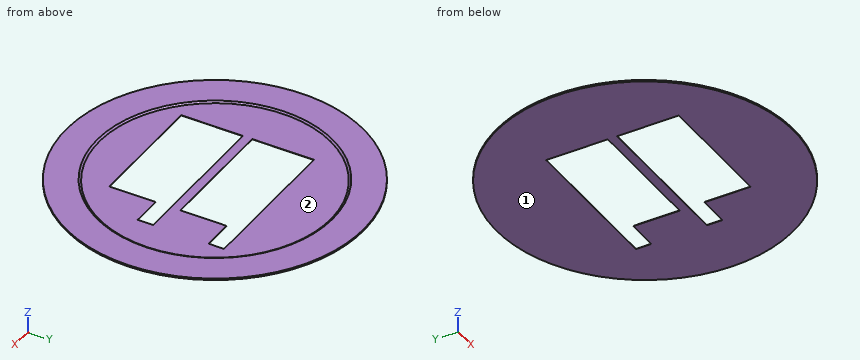
```python
from build123d import *

# Parameters (mm, degrees)
SKETCH3_W          = 40
SKETCH3_H          = 20
SKETCH3_W_2        = 10
SKETCH3_H_2        = 5
CUT_EXTRUDE1_DEPTH = 69.156113896


with BuildPart() as part:
    # Sketch2 → Revolve1 (revolve)
    with BuildSketch(Plane.YZ, mode=Mode.PRIVATE) as revolve1_sk:
        Polygon((48.192820323, 0.5), (38.192820323, 0.5), (37.5, 0.1), (0, 0.1), (0, 0), (48.192820323, 0), align=None)
    revolve(revolve1_sk.sketch.rotate(Axis((0, 0, 0.1), (0, 0, -1)), 90), axis=Axis((0, 0, 0.1), (0, 0, -1)))

    # Sketch3 → Cut-Extrude1 (cut, through all)
    with BuildSketch(Plane.XY.offset(0.1)):
        with Locations((-2.605575449, 8.919047288)):
            Rectangle(SKETCH3_W, SKETCH3_H)
        with Locations((22.394424551, 16.419047288)):
            Rectangle(SKETCH3_W_2, SKETCH3_H_2)
        with Locations((-2.605575449, -14.080952712)):
            Rectangle(SKETCH3_W, SKETCH3_H)
        with Locations((22.394424551, -6.580952712)):
            Rectangle(SKETCH3_W_2, SKETCH3_H_2)
    extrude(amount=-CUT_EXTRUDE1_DEPTH, mode=Mode.SUBTRACT)


solid = part.part
```
The listing builds one solid part. Answer for the finished solid, in the listing's coordinates (mm). Face numbers are marked on the shaded views. Coordinates: 2 decimals unless noted, no trailing zeros. Loops run counter-clockwise (first coordinate to the right, second up) from the corner with the lowest first, then second, coordinate; pieces in that order, holes last. Notation, with made-up numbers: (4.5, -15.5) - (40.5, -15.5) arc R12 ccw to (40.5, -1.5) - close; hole circle Ø10 at (61.5, 24). An arc over 180 degrees is marked (long way). Use a Markdown table: item, result. Add a question column.
1) The mould has two halves that part along X. Classify the marked faces 1 and 2: released by +X, released by -X, zero draft, split by the parting line, or undercut.
2) The part is cut by section B-B, the plane x = -1. State how many separate pieces and enclosed holes the cut face has, and give its area (3 significant figures).
3) The part is cut by section A-A, the plane z = 0.35. Give the vertices of the cut face in (x, y), and give its area (3 significant figures).
4) Given pin 1 (22.5 mm diameter, centred on x = 9.5, y = 17, fed in from +Z), flat-ended and moving along its own axis, determine where the tip first touches the part or whether it passes through.
5) Find the intervals of material crossed by line 1 (X direction, y = -11, z = 0.15); line 2 (X direction, y = 27, z = 0.25); line 3 (Y direction, x = 0, z = 0.4), in increasing order.
Here are the results:
| question | item | result |
|---|---|---|
| 1 | face 1 | zero draft |
| 1 | face 2 | undercut |
| 2 | separate pieces | 3 |
| 2 | enclosed holes | 0 |
| 2 | area | 13.9 mm^2 |
| 3 | outline | circle Ø96.39 at (0, 0); hole circle Ø75.87 at (0, 0) |
| 3 | area | 2,780 mm^2 |
| 4 | pin 1 | stops at z = 0.1 |
| 5 | line 1 | x = -46.92 to -35.94, 35.94 to 46.92 |
| 5 | line 2 | x = -39.92 to -26.4, 26.4 to 39.92 |
| 5 | line 3 | y = -48.19 to -38.02, 38.02 to 48.19 |
